Design review of the part built by this model. Coordinates are the model's own, in mm. Face numbers are marked on the shaded views. A direction names the side the tool comes from. Coordinates: 2 decimals unless noted, no trailing zeros. Write each loop counter-clockwise with the first axis right and the second up, starting at its lowest first coordinate (ties: lowest second). Pieces come first, ordered by that corner, then holes. Notation, with made-up numbers: M 2.25,77.25 L 41.25,77.25 A17 ccw 41.25,96.25 Z; hole C -16,44.25 d11. An arc over 180 degrees is marked long. One line per question, with ' | ' between items.
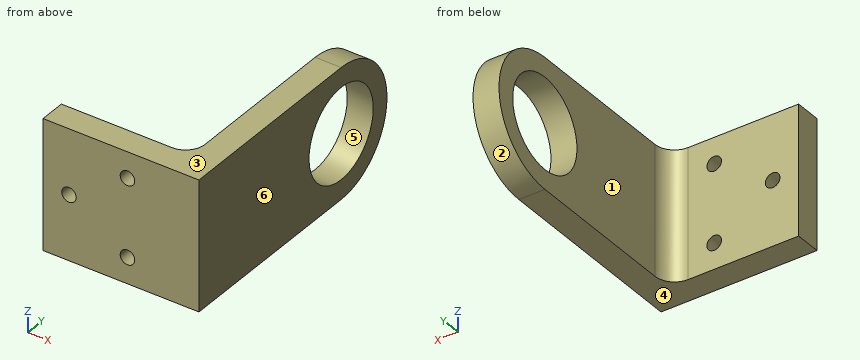
from build123d import *

# Parameters (mm, degrees)
SKETCH3_R           = 11.1125
BOSS_EXTRUDE1_DEPTH = 6.35
SKETCH5_W           = 31.75
SKETCH5_H           = 6.35
BOSS_EXTRUDE2_DEPTH = 38.1
FILLET1_R           = 4.7625
SKETCH6_R           = 1.777000002
CUT_EXTRUDE1_DEPTH  = 7.35


with BuildPart() as part:
    # Sketch3 → Boss-Extrude1 (new body)
    with BuildSketch(Plane(origin=(0, 0, 0), x_dir=(0, 0, -1), z_dir=(1, 0, 0))):
        with BuildLine():
            Line((0, 0), (31.75, 0))
            Line((31.75, 0), (31.75, 42.8625))
            ThreePointArc((31.75, 42.8625), (15.875, 58.7375), (0, 42.8625))
            Line((0, 42.8625), (0, 0))
        make_face()
        with Locations((15.875, 42.8625)):
            Circle(SKETCH3_R, mode=Mode.SUBTRACT)
    extrude(amount=BOSS_EXTRUDE1_DEPTH)

    # Sketch5 → Boss-Extrude2 (add)
    with BuildSketch(Plane(origin=(6.35, 0, 0), x_dir=(0, 0, -1), z_dir=(1, 0, 0))):
        with Locations((15.875, -3.175)):
            Rectangle(SKETCH5_W, SKETCH5_H)
    extrude(amount=-BOSS_EXTRUDE2_DEPTH)

    # Fillet1
    fillet1_edges = [part.edges().sort_by_distance(p)[0] for p in [
        (0, 0, -15.875),
    ]]
    fillet(fillet1_edges, radius=FILLET1_R)

    # Sketch6 → Cut-Extrude1 (cut, through all)
    with BuildSketch(Plane(origin=(0, 0, 0), x_dir=(1, 0, 0), z_dir=(0, 1, 0))):
        with Locations((-11.1125, 6.35)):
            Circle(SKETCH6_R)
        with Locations((-25.4, 15.875)):
            Circle(SKETCH6_R)
        with Locations((-11.1125, 25.4)):
            Circle(SKETCH6_R)
    extrude(amount=-CUT_EXTRUDE1_DEPTH, mode=Mode.SUBTRACT)


solid = part.part
1. Draft analysis for pull direction Z (two halves, no side actions). For the marked faces 3, 4, 5 and 6, state which applies: pulls with the +Z half, pulls with the -Z half, needs draft (parallel to the pull), parting line crosses it, or undercut.
Answer sheet:
face 3: pulls with the +Z half | face 4: pulls with the -Z half | face 5: undercut | face 6: needs draft
2. Take a section at C-C (y = 50.5). Write out the cut boundary in (x, z).
Answer sheet:
outline: M 0,-29.79 L 6.35,-29.79 L 6.35,-23.95 L 0,-23.95 Z; M 0,-7.8 L 6.35,-7.8 L 6.35,-1.96 L 0,-1.96 Z
3. To check wall thickness, follow line 1 along X through (y, z) = (29.5, -24); line 2 along Y through (x, z) = (-22.5, -21); line 3 along Z through (x, y) = (4, 40.5). State the ranges of each line that lie inside material, in increasing order. Write a range as [from, to].
Answer sheet:
line 1: [0, 6.35] | line 2: [-6.35, 0] | line 3: [-31.75, -26.73], [-5.02, 0]
4. Insertion check: pin 1 Ø3 at (x, z) = (-11.11, -6.35) entering from -Y; pin 2 Ø4 at (x, z) = (-20.5, -27.5) entering from +Y; pin 3 Ø9.5 at (y, z) = (24.5, -20.5) entering from -X. Each pin has a flat end and moves straight along its axis. Give the tip position at first contact, or say it passes through.
Answer sheet:
pin 1: through | pin 2: y = 0 | pin 3: x = 0
5. Take a section at A-A (z = -5.5). Count the separate pieces of the cut face and the enclosed holes in it, then the cut area to 3 significant figures.
Answer sheet:
separate pieces: 3 | enclosed holes: 0 | area: 525 mm^2
6. Take a section at B-B (x = -25.4). Write out the cut boundary in (y, z), then the cut area to 3 significant figures.
Answer sheet:
outline: M -6.35,-31.75 L 0,-31.75 L 0,-17.65 L -6.35,-17.65 Z; M -6.35,-14.1 L 0,-14.1 L 0,0 L -6.35,0 Z | area: 179 mm^2
7. Tool access review of the marked faces 1 and 2: name each direction out of +Z, -Z, +X, -X, +Y, -Y from which nothing blocks a thin tool from reaching the whole face with its end or side.
Answer sheet:
face 1: +Z, -Z, -X, +Y | face 2: +X, -X, +Y
